from build123d import *

# Parameters (mm, degrees)
CYLINDER729_R     = 20
CYLINDER729_DEPTH = 5
CYLINDER728_R     = 30
CYLINDER728_DEPTH = 5


with BuildPart() as cylinder799:
    # Cylinder729 → Cylinder729 (new body)
    with BuildSketch(Plane(origin=(0, -8, 28), x_dir=(1, 0, 0), z_dir=(0, 0, 1))):
        Circle(CYLINDER729_R)
    extrude(amount=CYLINDER729_DEPTH)


with BuildPart() as bearing:
    # Cylinder728 → Cylinder728 (new body)
    with BuildSketch(Plane(origin=(0, -8, 28), x_dir=(1, 0, 0), z_dir=(0, 0, 1))):
        Circle(CYLINDER728_R)
    extrude(amount=CYLINDER728_DEPTH)

    # Cut012035013: cut Cylinder799
    add(cylinder799.part, mode=Mode.SUBTRACT)


with BuildPart() as bearing_1:
    # Cut012035013 placement: moved
    add(bearing.part.moved(Location((0, 0, 4))))


solid = bearing_1.part
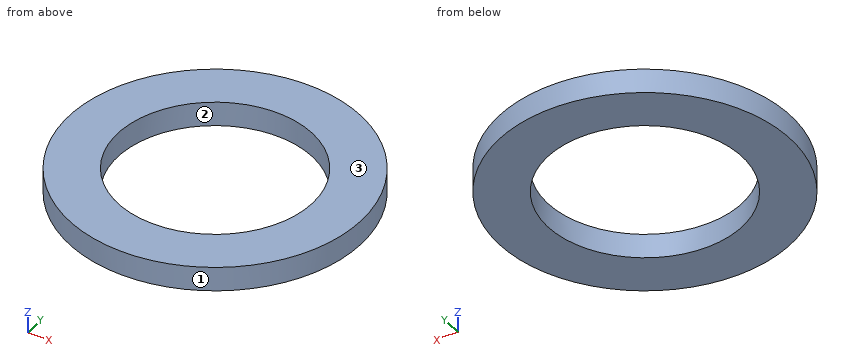
Source: CAD feature listing. Evaluate the final solid. Frame: model axes, mm. Face numbers are marked on the shaded views. Coordinates: 2 decimals unless noted, no trailing zeros. Order: outer loops, then holes, each group sorted by start corner. A loop starts at its lowest first (then second) coordinate and runs counter-clockwise, first axis right, second up.
Item 1: Cut plane A-A (y = -8). Return loops of the section in (x, z).
Output values:
outline: (-30, 32) - (-20, 32) - (-20, 37) - (-30, 37) - close; (20, 32) - (30, 32) - (30, 37) - (20, 37) - close
Item 2: Cut plane C-C (z = 33.3). Return loops of the section in (x, y), plus the area to 3 significant figures.
Output values:
outline: circle Ø60 at (0, -8); hole circle Ø40 at (0, -8)
area: 1,570 mm2
Item 3: Material intervals for line 1 (Y direction, x = 0, z = 33.1); line 2 (Y direction, x = -8, z = 32.95); line 3 (X direction, y = 4.5, z = 32.8), sorted ascending.
Output values:
line 1: y = -38 to -28, 12 to 22
line 2: y = -36.91 to -26.33, 10.33 to 20.91
line 3: x = -27.27 to -15.61, 15.61 to 27.27
Item 4: Pull-direction query (Y, two-part tool) for the marked faces 1, 2 and 3; classes: pulls with the +Y half, pulls with the -Y half, needs draft (parallel to the pull), parting line crosses it, or undercut.
Output values:
face 1: parting line crosses it
face 2: undercut
face 3: needs draft
Item 5: Cut plane B-B (x = 0). Return loops of the section in (y, z), plus the area to 3 significant figures.
Output values:
outline: (-38, 32) - (-28, 32) - (-28, 37) - (-38, 37) - close; (12, 32) - (22, 32) - (22, 37) - (12, 37) - close
area: 100 mm2
Item 6: First-contact query: P1, Ø1.5, axis at x = 4, z = 36, coming from the -Y side; P2, Ø3, axis at y = 4, z = 35.5, coming from the -X side; P3, Ø2, axis at x = -5, z = 36, coming from the +Y side. Flat tips, straight axial feed; report the tip coordinate or a pass-through.
Output values:
P1: stops at y = -37.82
P2: stops at x = -28.1
P3: stops at y = 21.73
